Check sheet for the drawn part. Datum: minimum x, y, z corner. Units: mm. A direction names the side the tool comes from. Coordinates: 2 decimals unless noted, no trailing zeros. Order: outer loops, then holes, each group sorted by start corner. A loop starts at its lowest first (then second) coordinate and runs counter-clockwise, first axis right, second up. Notation, with made-up numbers: M 7,38.5 L 61,38.5 A15 ccw 61,56.5 Z; hole C 72,-20 d10. An arc over 180 degrees is marked long. Return JSON: item names as keys, results as strings. Group by question number.
Q1. Thickness scan on probe 1 along Z at (x, y) = (3, 0.9); probe 2 along X at (y, z) = (0.9, 3); probe 3 along Y at (x, z) = (7.55, 15). Record the ranges inside material, lowest first.
Q2. Section check D-D, the plane z = 7. Enter the section's corners in (x, y).
Q3. Access from +Z, -Z, +X, -X, +Y, -Y to the whole of each face (thin tool, end or side, straight path). Record for the marked faces 5 and 6.
Q4. Go/stop test with flat-tipped pins: pin 1 Ø2 at (y, z) = (4, 10) entering from -X; pin 2 Ø1.6 at (x, z) = (4, 7) entering from +Y. Record where each tip stops, or that it passes through.
Q5. Section check A-A, the plane x = 3. Enter the section's corners in (y, z).
Q6. Section check C-C, the plane y = 1. Enter the section's corners in (x, z), then the cut area to 3 significant figures.
Q7. Section check B-B, the plane z = 3. Enter the section's corners in (x, y), then the cut area to 3 significant figures.
Q8. Mould release check, pull along X, two halves, no side actions. Record for the marked faces 1, 2, 3 and 4: pulls with the +X half, pulls with the -X half, needs draft (parallel to the pull), parting line crosses it, or undercut.
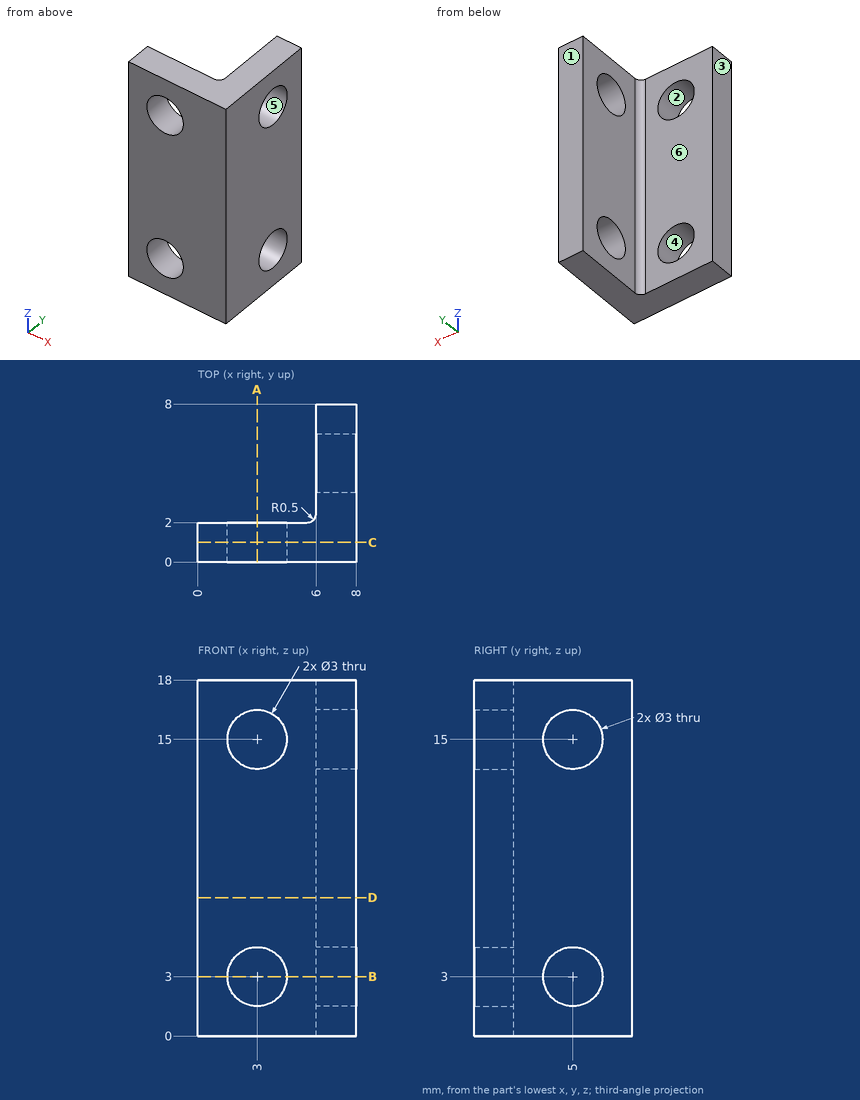
Numbers:
{
 "1": {"probe 1": "z = 0 to 1.5, 4.5 to 13.5, 16.5 to 18", "probe 2": "x = 0 to 1.5, 4.5 to 8", "probe 3": "y = 0 to 3.5, 6.5 to 8"},
 "2": {"outline": "M 0,0 L 8,0 L 8,8 L 6,8 L 6,2.5 A0.5 cw 5.5,2 L 0,2 Z"},
 "3": {"face 5": "+X, -X", "face 6": "+Z, -Z, -X, +Y"},
 "4": {"pin 1": "stops at x = 6", "pin 2": "stops at y = 2"},
 "5": {"outline": "M 0,0 L 2,0 L 2,1.5 L 0,1.5 Z; M 0,4.5 L 2,4.5 L 2,13.5 L 0,13.5 Z; M 0,16.5 L 2,16.5 L 2,18 L 0,18 Z"},
 "6": {"outline": "M 0,0 L 8,0 L 8,18 L 0,18 Z; hole C 3,3 d3; hole C 3,15 d3", "area": "130 mm2"},
 "7": {"outline": "M 0,0 L 1.5,0 L 1.5,2 L 0,2 Z; M 4.5,0 L 8,0 L 8,3.5 L 6,3.5 L 6,2.5 A0.5 cw 5.5,2 L 4.5,2 Z; M 6,6.5 L 8,6.5 L 8,8 L 6,8 Z", "area": "16.1 mm2"},
 "8": {"face 1": "needs draft", "face 2": "undercut", "face 3": "pulls with the -X half", "face 4": "undercut"}
}
